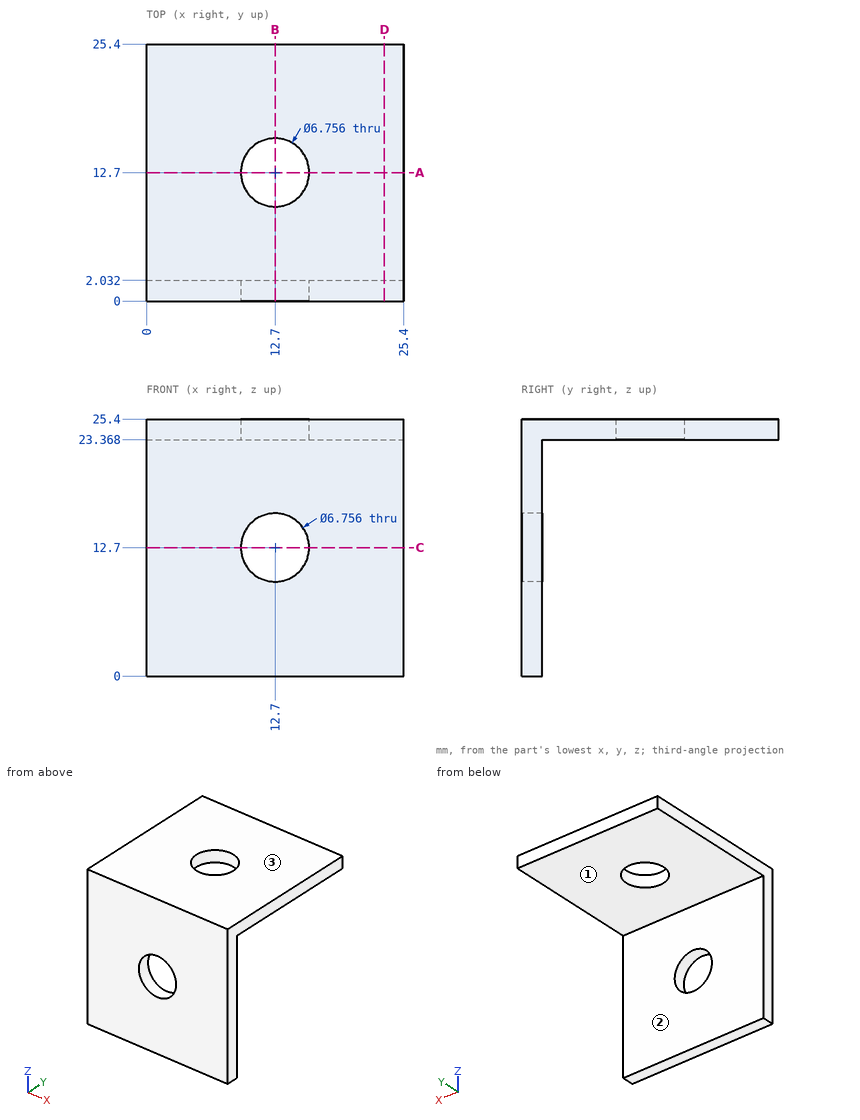
Geometry: see drawing. Coordinates: mm, zero at the bounding-box minimum. Coordinates: 2 decimals unless noted, no trailing zeros. Order: outer loops, then holes, each group sorted by start corner. A loop starts at its lowest first (then second) coordinate and runs counter-clockwise, first axis right, second up. Notation, with made-up numbers: M 85.25,-18.75 L 122.25,-18.75 A12 ccw 122.25,0.25 Z; hole C 51,-14.75 d7. An arc over 180 degrees is marked long. Write item = value, one per line. Start each with the question number.
(1) Section D-D on x = 23.5. Output: boundary loops of the cut face in (y, z).
(2) Pull-direction query (Z, two-part tool) for the marked faces 1, 2 and 3; classes: released by +Z, released by -Z, zero draft, split by the parting line, or undercut.
(3) Section C-C on z = 12.7. Output: boundary loops of the cut face in (x, y).
(4) First-contact query: P1, Ø10, axis at y = 14, z = 16.5, coming from the -X side; P2, Ø11, axis at x = 12.7, z = 12.7, coming from the +Y side; P3, Ø3, axis at x = 18.5, y = 21, coming from the -Z side; P4, Ø11, axis at x = 12.7, y = 12.7, coming from the +Z side. Flat tips, straight axial feed; report the tip coordinate or a pass-through.
(5) Section A-A on y = 12.7. Output: boundary loops of the cut face in (x, z).
(6) Line query: line 1 along Y through (x, z) = (12.7, 24.15); line 2 along Z through (x, y) = (12.5, 1.25); line 3 along Y through (x, z) = (7, 5). Output: solid intervals per line, ascending. Write a range as [from, to].
(7) Section B-B on x = 12.7. Output: boundary loops of the cut face in (y, z).
Result set:
q1.outline = M 0,0 L 2.03,0 L 2.03,23.37 L 25.4,23.37 L 25.4,25.4 L 0,25.4 Z
q2.face_1 = released by -Z
q2.face_2 = zero draft
q2.face_3 = released by +Z
q3.outline = M 0,0 L 9.32,0 L 9.32,2.03 L 0,2.03 Z; M 16.08,0 L 25.4,0 L 25.4,2.03 L 16.08,2.03 Z
q4.P1 = through
q4.P2 = 2.03
q4.P3 = 23.37
q4.P4 = 25.4
q5.outline = M 0,23.37 L 9.32,23.37 L 9.32,25.4 L 0,25.4 Z; M 16.08,23.37 L 25.4,23.37 L 25.4,25.4 L 16.08,25.4 Z
q6.line_1 = [0, 9.32], [16.08, 25.4]
q6.line_2 = [0, 9.33], [16.07, 25.4]
q6.line_3 = [0, 2.03]
q7.outline = M 0,0 L 2.03,0 L 2.03,9.32 L 0,9.32 Z; M 0,16.08 L 2.03,16.08 L 2.03,23.37 L 9.32,23.37 L 9.32,25.4 L 0,25.4 Z; M 16.08,23.37 L 25.4,23.37 L 25.4,25.4 L 16.08,25.4 Z
